```python
from build123d import *

# Parameters (mm, degrees)
SKETCH1_W           = 65
SKETCH1_H           = 65
BOSS_EXTRUDE1_DEPTH = 4
SKETCH2_R           = 11.25
CUT_EXTRUDE1_DEPTH  = 4
SKETCH3_W           = 10
SKETCH3_H           = 4
SKETCH3_W_2         = 15
CUT_EXTRUDE2_DEPTH  = 4
SKETCH5_W           = 4
SKETCH5_H           = 6
SKETCH5_H_2         = 15
CUT_EXTRUDE3_DEPTH  = 4
SKETCH6_R           = 1.55
SKETCH6_R_2         = 4
CUT_EXTRUDE4_DEPTH  = 4
BOSS_EXTRUDE3_DEPTH = 4
CUT_EXTRUDE6_DEPTH  = 4


with BuildPart() as part:
    # Sketch1 → Boss-Extrude1 (new body)
    with BuildSketch(Plane(origin=(0, 0, 0), x_dir=(0, 0, -1), z_dir=(1, 0, 0))):
        with Locations((32.5, 32.5)):
            Rectangle(SKETCH1_W, SKETCH1_H)
    extrude(amount=BOSS_EXTRUDE1_DEPTH)

    # Sketch2 → Cut-Extrude1 (cut)
    with BuildSketch(Plane(origin=(4, 0, 0), x_dir=(0, 0, -1), z_dir=(1, 0, 0))):
        with Locations((32.5, 32.5)):
            Circle(SKETCH2_R)
    extrude(amount=-CUT_EXTRUDE1_DEPTH, mode=Mode.SUBTRACT)

    # Sketch3 → Cut-Extrude2 (cut)
    with BuildSketch(Plane(origin=(4, 0, 0), x_dir=(0, 0, -1), z_dir=(1, 0, 0))):
        with Locations((5, 63)):
            Rectangle(SKETCH3_W, SKETCH3_H)
        with Locations((32.5, 63)):
            Rectangle(SKETCH3_W_2, SKETCH3_H)
        with Locations((60, 63)):
            Rectangle(SKETCH3_W, SKETCH3_H)
        with Locations((60, 2)):
            Rectangle(SKETCH3_W, SKETCH3_H)
        with Locations((32.5, 2)):
            Rectangle(SKETCH3_W_2, SKETCH3_H)
        with Locations((5, 2)):
            Rectangle(SKETCH3_W, SKETCH3_H)
    extrude(amount=-CUT_EXTRUDE2_DEPTH, mode=Mode.SUBTRACT)

    # Sketch5 → Cut-Extrude3 (cut)
    with BuildSketch(Plane(origin=(4, 0, 0), x_dir=(0, 0, -1), z_dir=(1, 0, 0))):
        with Locations((2, 58)):
            Rectangle(SKETCH5_W, SKETCH5_H)
        with Locations((2, 32.5)):
            Rectangle(SKETCH5_W, SKETCH5_H_2)
        with Locations((2, 7)):
            Rectangle(SKETCH5_W, SKETCH5_H)
        with Locations((63, 7)):
            Rectangle(SKETCH5_W, SKETCH5_H)
        with Locations((63, 32.5)):
            Rectangle(SKETCH5_W, SKETCH5_H_2)
        with Locations((63, 58)):
            Rectangle(SKETCH5_W, SKETCH5_H)
    extrude(amount=-CUT_EXTRUDE3_DEPTH, mode=Mode.SUBTRACT)

    # Sketch6 → Cut-Extrude4 (cut)
    with BuildSketch(Plane(origin=(4, 0, 0), x_dir=(0, 0, -1), z_dir=(1, 0, 0))):
        with Locations((7.5, 37.5)):
            Circle(SKETCH6_R)
        with Locations((17.5, 37.5)):
            Circle(SKETCH6_R)
        with Locations((17.5, 27.5)):
            Circle(SKETCH6_R)
        with Locations((12.5, 32.5)):
            Circle(SKETCH6_R_2)
        with Locations((7.5, 27.5)):
            Circle(SKETCH6_R)
        with Locations((52.5, 32.5)):
            Circle(SKETCH6_R_2)
        with Locations((47.5, 27.5)):
            Circle(SKETCH6_R)
        with Locations((47.5, 37.5)):
            Circle(SKETCH6_R)
        with Locations((57.5, 37.5)):
            Circle(SKETCH6_R)
        with Locations((57.5, 27.5)):
            Circle(SKETCH6_R)
    extrude(amount=-CUT_EXTRUDE4_DEPTH, mode=Mode.SUBTRACT)

    # Sketch12 → Boss-Extrude3 (add)
    with BuildSketch(Plane(origin=(4, 0, 0), x_dir=(0, 0, -1), z_dir=(1, 0, 0))):
        with BuildLine():
            ThreePointArc((4, 67), (32.5, 68.351492738), (61, 67))
            Line((61, 67), (61, 61))
            Line((61, 61), (55, 61))
            Line((55, 61), (55, 65))
            Line((55, 65), (40, 65))
            Line((40, 65), (40, 61))
            Line((40, 61), (25, 61))
            Line((25, 61), (25, 65))
            Line((25, 65), (10, 65))
            Line((10, 65), (10, 61))
            Line((10, 61), (4, 61))
            Line((4, 61), (4, 67))
        make_face()
    extrude(amount=-BOSS_EXTRUDE3_DEPTH)

    # Sketch11 → Cut-Extrude6 (cut)
    with BuildSketch(Plane(origin=(4, 0, 0), x_dir=(0, 0, -1), z_dir=(1, 0, 0))):
        with BuildLine():
            Line((20.5, 74.592318289), (20.5, 61.291011979))
            ThreePointArc((20.5, 61.291011979), (32.5, 49.291011979), (44.5, 61.291011979))
            Line((44.5, 61.291011979), (44.5, 74.592318289))
            Line((44.5, 74.592318289), (20.5, 74.592318289))
        make_face()
    extrude(amount=-CUT_EXTRUDE6_DEPTH, mode=Mode.SUBTRACT)


solid = part.part
```
Geometry check sheet. Reference: the model listing, model coordinates, mm. A direction names the side the tool comes from. Coordinates: 2 decimals unless noted, no trailing zeros. Order: outer loops, then holes, each group sorted by start corner. A loop starts at its lowest first (then second) coordinate and runs counter-clockwise, first axis right, second up. Notation, with made-up numbers: (11.25, 77.25) - (48.25, 77.25) arc R12 ccw to (48.25, 98.25) - close; hole circle Ø9 at (81, 53.5). An arc over 180 degrees is marked (long way). Use one line per item in the form item = value.
1. Scan lines: line 1 (Y direction, x = 1.55, z = -47.5); line 2 (Z direction, x = 3.55, y = 57); line 3 (Z direction, x = 2.35, y = 9). Record each from-to range of solid material in increasing order.
Here are the results:
line_1 = 0 to 25.95, 29.05 to 35.95, 39.05 to 67.98
line_2 = -61 to -43.71, -21.29 to -4
line_3 = -61 to -4
2. Section check B-B (z = -47.5). Record the boundary of the cut face in (x, y).
Here are the results:
outline = (0, 0) - (4, 0) - (4, 25.95) - (0, 25.95) - close; (0, 29.05) - (4, 29.05) - (4, 35.95) - (0, 35.95) - close; (0, 39.05) - (4, 39.05) - (4, 67.98) - (0, 67.98) - close
3. Draft check along Y on faces 1 (the face through (2.028, 49.294, -32.236)), 2 (the face through (2, 2, -40)), 3 (the face through (2, 4, -32)), 4 (the face through (2.028, 36.906, -58.932)). Enter one of: pulls with the +Y half, pulls with the -Y half, needs draft (parallel to the pull), parting line crosses it, or undercut.
Here are the results:
face_1 = pulls with the +Y half
face_2 = needs draft
face_3 = pulls with the -Y half
face_4 = undercut
4. Section check C-C (y = 58). Record the boundary of the cut face in (x, z), then the cut area to 3 significant figures.
Here are the results:
outline = (0, -61) - (4, -61) - (4, -44.04) - (0, -44.04) - close; (0, -20.96) - (4, -20.96) - (4, -4) - (0, -4) - close
area = 136 mm²
5. Gauge pin test, flat ends, axial feed: pin 1 (1.2 mm diameter, centred on x = 1.5, y = 7, fed in from -Z); pin 2 (2 mm diameter, centred on x = 1.5, z = -36, fed in from -Y); pin 3 (2 mm diameter, centred on x = 1.5, z = -1.5, fed in from +Y). Record the tip position at first contact, or that the pin passes through.
Here are the results:
pin_1 = -61
pin_2 = 4
pin_3 = 55
6. Section check D-D (x = 2.05). State how many separate pieces and enclosed holes the cut face has, then the cut area to 3 significant figures.
Here are the results:
separate_pieces = 1
enclosed_holes = 11
area = 3,050 mm²
7. Section check A-A (y = 32.5). Record the boundary of the cut face in (x, z), then the cut area to 3 significant figures.
Here are the results:
outline = (0, -61) - (4, -61) - (4, -56.5) - (0, -56.5) - close; (0, -48.5) - (4, -48.5) - (4, -43.75) - (0, -43.75) - close; (0, -21.25) - (4, -21.25) - (4, -16.5) - (0, -16.5) - close; (0, -8.5) - (4, -8.5) - (4, -4) - (0, -4) - close
area = 74.0 mm²
8. Access from +Z, -Z, +X, -X, +Y, -Y to the whole of each face (thin tool, end or side, straight path). Record for faces 5 (the face through (2, 10, -63)), 6 (the face through (2, 65, -20.5)), 7 (the face through (2, 55, -2)).
Here are the results:
face_5 = -Z, +X, -X, -Y
face_6 = +X, -X, +Y
face_7 = +Z, +X, -X, +Y
